Input: part model. Units: mm. Frame: model coordinates. A direction names the side the tool comes from. Round coordinates to 2 decimals unless told otherwise and drop trailing zeros. Loops run counter-clockwise (first coordinate to the right, second up) from the corner with the lowest first, then second, coordinate; pieces in that order, holes last. Notation, with made-up numbers: M 64.5,76.5 L 80.5,76.5 A16 cw 80.5,89.5 Z; hole C -16,26.25 d6. An arc over 180 degrees is marked long. Put each result on its own line as item: value. Start each with the question number.
1) Section B-B on x = 4. Output: boundary loops of the cut face in (y, z).
2) Pin query (flat end, axial travel): pin 1 (2.5 mm diameter, centred on x = 11, y = -19, fed in from +Z); pin 2 (6 mm diameter, centred on y = -18.5, z = -7.5, fed in from +X); pin 3 (2 mm diameter, centred on y = -11, z = -8.5, fed in from -X). Return the tip coordinate at first contact, or that it passes through.
3) Section C-C on z = -1.25. Output: boundary loops of the cut face in (x, y), plus the area to 3 significant figures.
4) Section A-A on y = -30. Output: boundary loops of the cut face in (x, z), plus the area to 3 significant figures.
5) Line query: probe 1 along X at (y, z) = (-22, -5.75); probe 2 along Z at (x, y) = (5.5, -23); probe 3 along X at (y, z) = (-16, 2.5). Output: solid intervals per line, ascending.
6) Reachability of faces 1 (the face through (-3.009, -8, -8)), 2 (the face through (-12.202, -23.265, -5.474)), 3 (the face through (-21.933, -20.314, 15.131)), 4 (the face through (9, -8, -5.39)), 5 (the face through (-6.509, -25, 8)) from +Z, -Z, +X, -X, +Y, -Y: full face, straight path, thin tool, end or side. Return the list, or none.
7) Section D-D on x = -8.5. Output: boundary loops of the cut face in (y, z), plus the area to 3 significant figures.
8) Draft query along Y for faces 6 (the face through (-12, 0, 0)), 7 (the face through (12.491, -8, 5)), 8 (the face through (0.796, -28.513, 15.131)). Return one class per face: +Y half, -Y half, draft (parallel to the pull), parting line (faces both ways), or undercut.
from build123d import *

# Parameters (mm, degrees)
F0_W      = 34
F0_H      = 28
F1_DEPTH  = 34
F3_R      = 1.5
F4_DEPTH  = 12
F5_W      = 8
F5_H      = 6
F6_DEPTH  = 17
F2_R      = 1.5
F7_DEPTH  = 28.001
F8_W      = 23
F8_H      = 3
F9_DEPTH  = 4
F10_W     = 15
F10_H     = 11
F11_DEPTH = 17.001
F12_W     = 18
F12_H     = 3
F13_DEPTH = 16
F14_W     = 18
F14_H     = 3
F15_DEPTH = 16
F16_R     = 10
F17_R     = 2
F18_DEPTH = 25
F19_R     = 1


with BuildPart() as f1:
    # F0 (on Front) → F1 (new body)
    with BuildSketch(Plane.XZ):
        with Locations((0.991450157, 2.6100003274)):
            Rectangle(F0_W, F0_H)
    extrude(amount=F1_DEPTH)

    # F3 (on face) → F4 (cut)
    with BuildSketch(Plane(origin=(0, 0, -11.3899996726), x_dir=(1, 0, 0), z_dir=(0, 0, -1))):
        with Locations((-13.008549843, 22)):
            Circle(F3_R)
        with Locations((14.991450157, 22)):
            Circle(F3_R)
    extrude(amount=-F4_DEPTH, mode=Mode.SUBTRACT)

    # F5 (on face) → F6 (cut)
    with BuildSketch(Plane(origin=(0, 0, 0), x_dir=(-1, 0, 0), z_dir=(0, 1, 0))):
        Polygon((10.508549843, 16.6100003274), (-12.491450157, 16.6100003274), (-12.491450157, -5.3899996726), (-4.991450157, -5.3899996726), (3.008549843, -5.3899996726), (10.508549843, -5.3899996726), align=None)
        with Locations((-0.991450157, -8.3899996726)):
            Rectangle(F5_W, F5_H)
    extrude(amount=-F6_DEPTH, mode=Mode.SUBTRACT)

    # F2 (on face) → F7 (cut, through all)
    with BuildSketch(Plane.XY.offset(16.6100003274)):
        with Locations((0.991450157, -30)):
            Circle(F2_R)
    extrude(amount=-F7_DEPTH, mode=Mode.SUBTRACT)

    # F8 (on face) → F9 (cut)
    with BuildSketch(Plane(origin=(0, -17, 0), x_dir=(-1, 0, 0), z_dir=(0, 1, 0))):
        with Locations((-0.991450157, 15.1100003274)):
            Rectangle(F8_W, F8_H)
    extrude(amount=-F9_DEPTH, mode=Mode.SUBTRACT)

    # F10 (on face) → F11 (cut, through all)
    with BuildSketch(Plane(origin=(0, -17, 0), x_dir=(-1, 0, 0), z_dir=(0, 1, 0))):
        with Locations((-0.991450157, 8.1100003274)):
            Rectangle(F10_W, F10_H)
    extrude(amount=-F11_DEPTH, mode=Mode.SUBTRACT)

    # F12 (on face) → F13 (join)
    with BuildSketch(Plane(origin=(-16.008549843, 0, 0), x_dir=(0, -1, 0), z_dir=(-1, 0, 0))):
        with Locations((25, 15.1100003274)):
            Rectangle(F12_W, F12_H)
    extrude(amount=F13_DEPTH)

    # F14 (on face) → F15 (join)
    with BuildSketch(Plane.YZ.offset(17.991450157)):
        with Locations((-25, 15.1100003274)):
            Rectangle(F14_W, F14_H)
    extrude(amount=F15_DEPTH)

    # F16
    f16_edges = [f1.edges().sort_by_distance(p)[0] for p in [
        (33.99145, -16, 15.11),
        (-32.00855, -16, 15.11),
    ]]
    fillet(f16_edges, radius=F16_R)

    # F17 (on face) → F18 (cut)
    with BuildSketch(Plane.XY.offset(16.6100003274)):
        with Locations((-23.008549843, -22)):
            Circle(F17_R)
        with Locations((24.991450157, -22)):
            Circle(F17_R)
        with BuildLine():
            Line((-16.008549843, -22.7352958173), (-16.008549843, -16))
            Line((-16.008549843, -16), (-22.008549843, -16))
            ThreePointArc((-22.008549843, -16), (-22.4260025255, -16.0087171365), (-22.8427274097, -16.0348533484))
            ThreePointArc((-22.8427274097, -16.0348533484), (-18.1144410308, -18.0477066054), (-16.008549843, -22.7352958173))
        make_face()
        with BuildLine():
            Line((18.007015779, -16), (18.1666726931, -21.9172614151))
            ThreePointArc((18.1666726931, -21.9172614151), (19.839883731, -17.7388207651), (23.991450157, -16))
            Line((23.991450157, -16), (18.007015779, -16))
        make_face()
    extrude(amount=-F18_DEPTH, mode=Mode.SUBTRACT)

    # F19
    f19_edges = [f1.edges().sort_by_distance(p)[0] for p in [
        (-16.00855, -17, -11.39),
        (17.99145, -17, -11.39),
        (4.99145, -8.5, -5.39),
        (-3.00855, -8.5, -5.39),
        (4.99145, -8.5, -11.39),
        (-3.00855, -8.5, -11.39),
        (12.49145, -10.5, 16.61),
        (-10.50855, -10.5, 16.61),
        (0.99145, -34, 2.61),
        (8.49145, -34, 8.11),
        (0.99145, -34, 13.61),
        (-6.50855, -34, 8.11),
        (-8.50855, -17, 13.61),
        (10.49145, -17, 13.61),
        (0.99145, -34, -11.39),
        (-9.50855, 0, -11.39),
        (11.49145, 0, -11.39),
    ]]
    fillet(f19_edges, radius=F19_R)


solid = f1.part
Geometry results:
1. outline: M -34,-10.39 A1 ccw -33,-11.39 L -17,-11.39 L -17,2.61 L -33,2.61 A1 ccw -34,1.61 Z; M -34,14.61 A1 ccw -33,13.61 L -21,13.61 L -21,16.61 L -34,16.61 Z
2. pin 1: stops at z = 13.61
2. pin 2: stops at x = 17.99
2. pin 3: stops at x = -16.01
3. outline: M -16.01,-34 L 17.99,-34 L 17.99,0 L 12.49,0 L 12.49,-17 L -10.51,-17 L -10.51,0 L -16.01,0 Z; hole C -13.01,-22 d3; hole C 0.99,-30 d3; hole C 14.99,-22 d3
3. area: 744 mm²
4. outline: M -32.01,13.61 L -16.01,13.61 L -16.01,-10.39 A1 ccw -15.01,-11.39 L -0.51,-11.39 L -0.51,2.61 L -6.51,2.61 L -6.51,13.61 L -0.51,13.61 L -0.51,16.61 L -32.01,16.61 Z; M 2.49,-11.39 L 16.99,-11.39 A1 ccw 17.99,-10.39 L 17.99,13.61 L 33.99,13.61 L 33.99,16.61 L 2.49,16.61 L 2.49,13.61 L 8.49,13.61 L 8.49,2.61 L 2.49,2.61 Z
4. area: 832 mm²
5. probe 1: x = -16.01 to -14.51, -11.51 to 13.49, 16.49 to 17.99
5. probe 2: z = -11.39 to 2.61, 13.61 to 16.61
5. probe 3: x = -16.01 to -10.51, 12.49 to 17.99
6. face 1: +Z, -Z, +Y
6. face 2: -Z
6. face 3: +Z, -Z
6. face 4: +Z, +Y
6. face 5: +Y, -Y
7. outline: M -34,-10.39 A1 ccw -33,-11.39 L -1,-11.39 A1 ccw 0,-10.39 L 0,-5.39 L -17,-5.39 L -17,12.61 A1 ccw -18,13.61 L -21,13.61 L -21,16.61 L -34,16.61 Z
7. area: 565 mm²
8. face 6: +Y half
8. face 7: draft
8. face 8: undercut
